Autodesk Inventor part; units mm, degrees
ref_plane "YZ Plane" through (0, 0, 0) normal (1, 0, 0) x (0, 1, 0)
ref_plane "XZ Plane" through (0, 0, 0) normal (0, 1, 0) x (-1, 0, 0)
ref_plane "XY Plane" through (0, 0, 0) normal (0, 0, 1) x (1, 0, 0)
sketch "Sketch1" plane through (0, 0, 0) normal (0, 1, 0) x (-1, 0, 0)
  line L0 (15, 0) -> (15, -15)
  line L1 (15, -15) -> (0, -15)
  line L2 (0, -15) -> (0, -12)
  line L3 (0, -12) -> (12, -12)
  line L4 (12, -12) -> (12, 0)
  line L5 (12, 0) -> (15, 0)
  point P0 (0, 0)
  dimension "d0" = 15
  dimension "d1" = 15
  dimension "d10" = 3
  dimension "d11" = 12
  dimension "d12" = 12
extrude "Extrusion1" add sketch "Sketch1" along normal blind 86
sketch "Sketch4" plane through (-12, 0, 0) normal (1, 0, 0) x (0, 0, -1)
  line L0 (0, 0) -> (0, 86)
  line L1 (12, 0) -> (12, 86)
  line L2 (0, 86) -> (12, 86)
  line L3 (12, 86) -> (12, 83)
  line L4 (12, 83) -> (0, 83)
  line L5 (0, 83) -> (0, 86)
  dimension "d13" = 3
extrude "Extrusion3" add sketch "Sketch4" along normal blind 3
sketch "Sketch6" plane through (-12, 0, -12) normal (0, 0, 1) x (1, 0, 0)
  line L0 (3, 86) -> (12, 86)
  line L1 (12, 86) -> (3, 86)
  line L2 (3, 86) -> (3, 83)
  line L3 (3, 83) -> (12, 83)
  line L4 (12, 83) -> (12, 86)
  point P0 (12, 0)
extrude "Extrusion4" add sketch "Sketch6" along normal blind 12
fillet "Fillet3" radius 2 7 edges at (-7.5, 86, -15) (-15, 86, -7.5) (-15, 43, -15) (0, 43, -15) (-7.5, 86, 0) (0, 86, -7.5) (-15, 43, 0)
sketch "Sketch11" plane through (0, 86, 0) normal (0, 1, 0) x (1, 0, 0)
  arc A0 (-15, 2) -> (-13, 0) centre (-13, 2) ccw
  line L0 (0, 10.8348) -> (0, 14)
  line L1 (-9, 9) -> (0, 9)
  line L2 (0, 9) -> (0, 10.8348)
  line L3 (-9, 15) -> (0, 15)
  line L4 (0, 15) -> (0, 9)
  line L5 (-9, 15) -> (-9, 9)
  line L6 (0, 0) -> (0, 13)
  point P0 (-13, 0)
  point P1 (0, 15)
extrude "Extrusion7" cut sketch "Sketch11" against normal blind 6
sketch "Sketch12" plane through (-12, 0, -12) normal (0, 0, 1) x (1, 0, 0)
  line L0 (12, 33) -> (21, 33) construction
  line L1 (3, 39) -> (12, 39)
  line L2 (12, 0) -> (12, 80)
  line L3 (3, 36) -> (12, 36)
  line L4 (3, 39) -> (3, 36)
extrude "Extrusion8" cut sketch "Sketch12" against normal through all
properties part number "DoosjeHoeken" material "ABS Plastic"
Model file for the job. Use its own axes, mm. A direction names the side the tool comes from. Give positions to 0.01 mm unless a question says otherwise; leave off trailing zeros. Loops run counter-clockwise (first coordinate to the right, second up) from the corner with the lowest first, then second, coordinate; pieces in that order, holes last. Notation, with made-up numbers: (55.25, -31) - (75.25, -31) arc R26 ccw to (75.25, -16) - close; hole circle Ø1 at (32.25, 40.5). An arc over 180 degrees is marked (long way). One line per item, written item: value. Start each with the question number.
1. Pull direction Y, two halves, no side cores. Call faces 4 (the flat face through (-5, 80, -14)), 5 (the flat face through (-9, 38, -13)), 6 (the flat face through (-5, 85, -9)), 7 (the flat face through (-5, 36, -13)): pulls with the +Y half, pulls with the -Y half, needs draft (parallel to the pull), parting line crosses it, or undercut.
2. Probe L1, parallel to Y at x = -2.25, z = -13; L2, parallel to Z at x = -8.75, y = 46.5; L3, parallel to X at y = 70.5, z = -1.75. List the from-to ranges inside material, lowest first. Write a range as from..to.
3. Slice it at D-D (z = -10). List the corners of the cut face in (x, y), plus the area to 3 significant figures.
4. Pin check, flat tips, straight feed: pin 1 (3.5 mm diameter, centred on x = -4, z = -13, fed in from +Y); pin 2 (0.9 mm diameter, centred on y = 37, z = -14, fed in from +X); pin 3 (6 mm diameter, centred on x = -5, z = -5, fed in from -Y). Stop position of each tip, or through.
5. Slice it at C-C (z = -6.5). List the corners of the cut face in (x, y).
6. Slice it at B-B (y = 43). List the corners of the cut face in (x, z).
7. Which spindle directions (+Z, -Z, +X, -X, +Y, -Y) get a long thin tool onto all of the face, cutting with end or side? Do faces 1 (the flat face through (-6, 41, -12)), 2 (the flat face through (-9, 84, -12)), 3 (the cylindrical face through (-0.6, 85.43, -4.56)). Say none if no direction does.
8. Slice it at A-A (x = -8). List the corners of the cut face in (y, z).
Solution:
1. face 4: pulls with the +Y half
1. face 5: undercut
1. face 6: needs draft
1. face 7: undercut
2. L1: y = 0..36, 39..80
2. L2: z = -15..-12
2. L3: x = -14.98..-12
3. outline: (-15, 0) - (-12, 0) - (-12, 83) - (-9, 83) - (-9, 86) - (-13, 86) arc R2 ccw to (-15, 84) - close
3. area: 266 mm^2
4. pin 1: stops at y = 80
4. pin 2: stops at x = -9
4. pin 3: stops at y = 83
5. outline: (-15, 0) - (-12, 0) - (-12, 83) - (0, 83) - (0, 84) arc R2 ccw to (-2, 86) - (-13, 86) arc R2 ccw to (-15, 84) - close
6. outline: (-15, -13) arc R2 ccw to (-13, -15) - (-2, -15) arc R2 ccw to (0, -13) - (0, -12) - (-12, -12) - (-12, 0) - (-13, 0) arc R2 ccw to (-15, -2) - close
7. face 1: +Z, +X, -Y
7. face 2: -Z, +X, +Y
7. face 3: +Z, -Z, +X, +Y
8. outline: (0, -15) - (36, -15) - (36, -12) - (0, -12) - close; (39, -15) - (80, -15) - (80, -12) - (39, -12) - close; (83, -9) - (86, -9) - (86, -2) arc R2 ccw to (84, 0) - (83, 0) - close
